Here's how the part is built. I have some questions about the finished solid (model axes, mm). A direction names the side the tool comes from. Round coordinates to 2 decimals unless told otherwise and drop trailing zeros. Loops run counter-clockwise (first coordinate to the right, second up) from the corner with the lowest first, then second, coordinate; pieces in that order, holes last. Notation, with made-up numbers: (-4.5, 47.25) -> (9.5, 47.25) arc R18 ccw to (9.5, 58.25) -> close; hole circle Ø10 at (69, 31.25). An arc over 180 degrees is marked (long way). Use one line per item in the form item = value. Start each with the question number.
Item 1: If we section it at D-D (y = -9): Write out the boundary of the cut face in (x, z) (3 decimals), then the cut area to 3 significant figures.
Item 2: If we section it at A-A (z = 6.35): Write out the boundary of the cut face in (x, y) (3 decimals), then the cut area to 3 significant figures.
Item 3: If I drill on L1, parallel to Y at x = 31, z = 5.25; L2, parallel to Y at x = -19.05, z = 5.5; L3, parallel to X at y = 6, z = 4.75 (3 decimals), over which ranges is the centre line in solid material (lowest first)? Write a range as [from, to].
Item 4: If we section it at B-B (x = -7.62): Write out the boundary of the cut face in (y, z), then the cut area to 3 significant figures.
Item 5: I'm going to push flat-ended pins straight in: pin 1 Ø6.5 at (x, z) = (29, 3.5) entering from -Y; pin 2 Ø8 at (x, y) = (-19.05, -34.925) entering from +Z; pin 3 Ø6.5 at (x, z) = (34.5, 3.5) entering from +Y; pin 4 Ø11.5 at (x, y) = (-19.05, 34.925) entering from +Z. Where does each tip first touch, or does it pass through?
Item 6: Thinking about a two-plate mould opening in Z: for faces 5 (the face through (41.275, -7, 6)), 6 (the face through (18, 11, 0)), 7 (the face through (12, 28, 12.7)), 8 (the face through (38.274, 6.519, 6.79)), which applies, released by +Z, released by -Z, zero draft, split by the parting line, or undercut?
Item 7: If we section it at C-C (y = 21): Write out the boundary of the cut face in (x, z) (3 decimals), then the cut area to 3 significant figures.
Item 8: For faces 1 (the face through (18, -27, 12.7)), 2 (the face through (26.035, 30, 6)), 3 (the face through (-22.5, -38.6, 5.1)), 4 (the face through (32, -12.7, 4)), which set-ups out of +Z, -Z, +X, -X, +Y, -Y let a thin tool reach every point of the face, with its end or its side?
```python
from build123d import *

# Parameters (mm, degrees)
SKETCH1_W               = 82.55
SKETCH1_H               = 88.9
EXTRUDE1_DEPTH          = 12.7
SKETCH2_R               = 27.1272
EXTRUDE2_DEPTH          = 62.973527615
SKETCH3_W               = 28.468633454
SKETCH3_H               = 1.016
EXTRUDE3_DEPTH          = 62.973527615
F_1_4_CLEARANCE_HOLE1_D = 6.7564
SKETCH10_W              = 15.24
SKETCH10_H              = 31.75
EXTRUDE4_DEPTH          = 62.973527707
FILLET1_R               = 3.175


with BuildPart() as part:
    # Sketch1 → Extrude1 (new body)
    with BuildSketch(Plane.XY):
        Rectangle(SKETCH1_W, SKETCH1_H)
    extrude(amount=EXTRUDE1_DEPTH)

    # Sketch2 → Extrude2 (cut, through all)
    with BuildSketch(Plane.XY.offset(12.7)):
        with Locations((-7.62, 0)):
            Circle(SKETCH2_R)
    extrude(amount=-EXTRUDE2_DEPTH, mode=Mode.SUBTRACT)

    # Sketch3 → Extrude3 (cut, through all)
    with BuildSketch(Plane.XY.offset(12.7)):
        with Locations((30.3911, 0)):
            Rectangle(SKETCH3_W, SKETCH3_H)
    extrude(amount=-EXTRUDE3_DEPTH, mode=Mode.SUBTRACT)

    # 1/4 Clearance Hole1 (through all)
    with Locations(Plane(origin=(34.925, 44.45, 6.35), x_dir=(0, 0, 1), z_dir=(0, 1, 0))):
        with Locations((0, 0)):
            Hole(F_1_4_CLEARANCE_HOLE1_D / 2)

    # Sketch9 → CSK for 3/8 Flat Head Machine Screw (100)1 (revolve, cut)
    with BuildSketch(Plane(origin=(-19.05, 34.925, 12.7), x_dir=(0, -1, 0), z_dir=(1, 0, 0))):
        Polygon((0, 0), (0, 14.459479155), (5.0419, 11.43), (5.0419, 3.88964634), (9.6774, 0), align=None)
    csk_for_3_8_flat_head_machine_screw_100 = revolve(axis=Axis((-19.05, 34.925, 19.05), (0, 0, -1)), mode=Mode.SUBTRACT)

    # Mirror1: CSK for 3/8 Flat Head Machine Screw (100)1 across plane
    add(csk_for_3_8_flat_head_machine_screw_100.mirror(Plane.ZX), mode=Mode.SUBTRACT)

    # Sketch10 → Extrude4 (cut, through all)
    with BuildSketch(Plane.XY.offset(12.7)):
        with Locations((33.655, 28.575)):
            Rectangle(SKETCH10_W, SKETCH10_H)
    extrude4 = extrude(amount=-EXTRUDE4_DEPTH, mode=Mode.SUBTRACT)

    # Mirror2: Extrude4 across plane
    add(extrude4.mirror(Plane.ZX), mode=Mode.SUBTRACT)

    # Fillet1
    fillet1_edges = [part.edges().sort_by_distance(p)[0] for p in [
        (26.035, -12.7, 6.35),
        (26.035, 12.7, 6.35),
    ]]
    fillet(fillet1_edges, radius=FILLET1_R)


solid = part.part
```
Values found:
q1.outline = (-41.275, 0) -> (-33.211, 0) -> (-33.211, 12.7) -> (-41.275, 12.7) -> close; (17.971, 0) -> (41.275, 0) -> (41.275, 12.7) -> (17.971, 12.7) -> close; hole circle Ø6.756 at (34.925, 6.35)
q1.area = 363 mm2
q2.outline = (-41.275, -44.45) -> (26.035, -44.45) -> (26.035, -15.875) arc R3.175 cw to (29.21, -12.7) -> (31.547, -12.7) -> (31.547, -0.508) -> (19.502, -0.508) arc R27.127 cw (long way) to (19.502, 0.508) -> (31.547, 0.508) -> (31.547, 12.7) -> (29.21, 12.7) arc R3.175 cw to (26.035, 15.875) -> (26.035, 44.45) -> (-41.275, 44.45) -> close; (38.303, -12.7) -> (41.275, -12.7) -> (41.275, -0.508) -> (38.303, -0.508) -> close; (38.303, 0.508) -> (41.275, 0.508) -> (41.275, 12.7) -> (38.303, 12.7) -> close; hole circle Ø10.084 at (-19.05, -34.925); hole circle Ø10.084 at (-19.05, 34.925)
q2.area = 3,720 mm2
q3.L1 = [-12.7, -0.51], [0.51, 12.7]
q3.L2 = [-44.45, -39.97], [-29.88, -24.6], [24.6, 29.88], [39.97, 44.45]
q3.L3 = [-41.275, -34.075], [18.835, 31.95], [37.9, 41.275]
q4.outline = (-44.45, 0) -> (-27.13, 0) -> (-27.13, 12.7) -> (-44.45, 12.7) -> close; (27.13, 0) -> (44.45, 0) -> (44.45, 12.7) -> (27.13, 12.7) -> close
q4.area = 440 mm2
q5.pin_1 = -44.45
q5.pin_2 = 0.64
q5.pin_3 = 12.7
q5.pin_4 = 9.4
q6.face_5 = zero draft
q6.face_6 = released by -Z
q6.face_7 = released by +Z
q6.face_8 = undercut
q7.outline = (-41.275, 0) -> (-24.792, 0) -> (-24.792, 12.7) -> (-41.275, 12.7) -> close; (9.552, 0) -> (26.035, 0) -> (26.035, 12.7) -> (9.552, 12.7) -> close
q7.area = 419 mm2
q8.face_1 = +Z, +X, -X, +Y, -Y
q8.face_2 = +Z, -Z, +X, +Y
q8.face_3 = +Z
q8.face_4 = +Z, -Z, +X, -Y
